Geometry check sheet. Reference: the model listing, model coordinates, mm. Face numbers are marked on the shaded views. A direction names the side the tool comes from. Round coordinates to 2 decimals unless told otherwise and drop trailing zeros. Write each loop counter-clockwise with the first axis right and the second up, starting at its lowest first coordinate (ties: lowest second). Pieces come first, ordered by that corner, then holes. Notation, with made-up numbers: (29.5, -1.5) -> (35.5, -1.5) arc R34 cw to (35.5, 32.5) -> close; hole circle Ø10 at (-38.5, 31). An arc over 180 degrees is marked (long way). One line per question, with ' | ' between items.
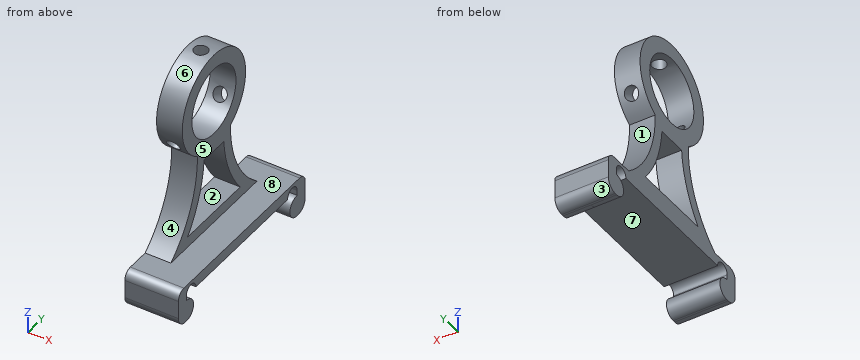
Autodesk Inventor part; units mm, degrees
ref_plane "Work Plane1" through (0, 0, 88) normal (0, 0, 1) x (1, 0, 0)
ref_plane "YZ Plane" through (0, 0, 0) normal (1, 0, 0) x (0, 1, 0)
ref_plane "XZ Plane" through (0, 0, 0) normal (0, 1, 0) x (-1, 0, 0)
sketch "Sketch1" plane through (0, 0, 0) normal (1, 0, 0) x (0, 1, 0)
  line L0 (-46, -7.5) -> (-46, 1)
  line L1 (-42, 5) -> (42, 5)
  line L2 (46, 1) -> (46, -7.5)
  line L3 (-41, -12.5) -> (-39.95, -12.5)
  line L4 (-40.25, -2.509) -> (-40.25, 0)
  line L5 (-40.25, 0) -> (40.25, 0)
  arc A0 (46, 1) -> (42, 5) centre (42, 1) ccw
  arc A1 (-42, 5) -> (-46, 1) centre (-42, 1) ccw
  arc A2 (40.25, 0) -> (33.25, 0) centre (36.75, 0) ccw
  arc A3 (-33.25, 0) -> (-40.25, 0) centre (-36.75, 0) ccw
  line L6 (40.25, 0) -> (40.25, -2.509)
  arc A4 (-39.95, -12.5) -> (-40.25, -2.509) centre (-39.95, -7.5) ccw
  arc A5 (-46, -7.5) -> (-41, -12.5) centre (-41, -7.5) ccw
  circle A6 centre (39.95, -7.5) radius 5
  line L7 (41, -12.5) -> (39.95, -12.5)
  arc A7 (41, -12.5) -> (46, -7.5) centre (41, -7.5) ccw
  circle A8 centre (0, 65) radius 16
  circle A9 centre (0, 65) radius 23
  arc A10 (-31.25, 5) -> (-12, 45.3786) centre (-61.9911, 44.4333) ccw
  arc A11 (12, 45.3786) -> (31.25, 5) centre (61.9911, 44.4333) ccw
  point P0 (0, 0)
  point P1 (-46, -12.5)
  point P2 (-46, 5)
  point P3 (46, 5)
  point P4 (46, -12.5)
  point P5 (0, 0)
  point P6 (-40.25, -1.2545)
  point P7 (40.25, -1.2545)
  point P8 (40.25, -2.509)
  point P9 (0, 5)
  dimension "d71" = 10
  dimension "d2" = 80.5
  dimension "d10" = 92
  dimension "d11" = 5
  dimension "d52" = 4
  dimension "d53" = 7
  dimension "d54" = 7
  dimension "d67" = 10
  dimension "d68" = 7.5
  dimension "d69" = 0.3
  dimension "d70" = 5
  dimension "d72" = 0.3
  dimension "d73" = 5
  dimension "d74" = 32
  dimension "d75" = 7
  dimension "d76" = 65
  dimension "d77" = 2
  dimension "d78" = 2
  dimension "d79" = 12
  dimension "d80" = 50
extrude "Extrusion1" add sketch "Sketch1" along normal mid plane 12 contours L0 A1 L1 A0 L2 A7 L7 A6 L6 A2 L5 A3 L4 A4 L3 A5 | A10 A9 A11 L1 | A9 | A6
sketch "Sketch7" plane through (6, 0, 0) normal (1, 0, 0) x (0, 0, -1)
  arc A0 (-45.3786, 12) -> (-5, 31.25) centre (-44.4333, 61.9911) ccw
  arc A1 (-5, -31.25) -> (-45.3786, -12) centre (-44.4333, -61.9911) ccw
  arc A2 (-45.3786, 12) -> (-45.3786, -12) centre (-65, 0) ccw
  line L0 (-45.3786, 12) -> (-45.3786, -12)
  arc A3 (-45.3786, 12) -> (-5, 31.25) centre (-44.4333, 61.9911) ccw
  line L1 (-5, 31.25) -> (-5, -31.25)
  line L2 (0, -33.25) -> (0, 33.25)
  arc A4 (-45.3786, 12) -> (-5, 31.25) centre (-44.4333, 61.9911) ccw
  arc A5 (-5, -31.25) -> (-45.3786, -12) centre (-44.4333, -61.9911) ccw
  arc A6 (-5, -31.25) -> (-45.3786, -12) centre (-44.4333, -61.9911) ccw
  arc A7 (-10, -19.1035) -> (-40.3786, -7.1407) centre (-44.4333, -61.9911) ccw
  line L3 (-40.3786, -7.1407) -> (-40.3786, 7.1407)
  arc A8 (-40.3786, 7.1407) -> (-10, 19.1035) centre (-44.4333, 61.9911) ccw
  line L4 (-10, 19.1035) -> (-10, -19.1035)
  point P0 (0, 0)
  dimension "d81" = 5
extrude "Extrusion4" cut sketch "Sketch7" against normal through all contours A7 L3 A8 L4
sketch "Sketch8" plane through (6, 0, 0) normal (1, 0, 0) x (0, 0, -1)
  line L0 (-40.3786, -7.1407) -> (-40.3786, 7.1407)
  arc A0 (-40.3786, 7.1407) -> (-10, 19.1035) centre (-44.4333, 61.9911) ccw
  line L1 (-10, 19.1035) -> (-10, -19.1035)
  arc A1 (-10, -19.1035) -> (-40.3786, -7.1407) centre (-44.4333, -61.9911) ccw
  arc A2 (0, -33.25) -> (0, -40.25) centre (0, -36.75) ccw
  line L2 (0, -33.25) -> (0, 33.25)
  arc A3 (0, 40.25) -> (0, 33.25) centre (0, 36.75) ccw
  line L3 (0, 40.25) -> (2.509, 40.25)
  arc A4 (2.509, 40.25) -> (12.5, 39.95) centre (7.5, 39.95) ccw
  line L4 (12.5, 39.95) -> (12.5, 41)
  arc A5 (12.5, 41) -> (7.5, 46) centre (7.5, 41) ccw
  line L5 (7.5, 46) -> (-1, 46)
  arc A6 (-1, 46) -> (-5, 42) centre (-1, 42) ccw
  line L6 (-5, 42) -> (-5, 31.25)
  arc A7 (-45.3786, 12) -> (-5, 31.25) centre (-44.4333, 61.9911) ccw
  arc A8 (-45.3786, 12) -> (-45.3786, -12) centre (-65, 0) ccw
  arc A9 (-5, -31.25) -> (-45.3786, -12) centre (-44.4333, -61.9911) ccw
  line L7 (-5, -31.25) -> (-5, -42)
  arc A10 (-5, -42) -> (-1, -46) centre (-1, -42) ccw
  line L8 (-1, -46) -> (7.5, -46)
  arc A11 (7.5, -46) -> (12.5, -41) centre (7.5, -41) ccw
  line L9 (12.5, -41) -> (12.5, -39.95)
  arc A12 (12.5, -39.95) -> (2.509, -40.25) centre (7.5, -39.95) ccw
  line L10 (2.509, -40.25) -> (0, -40.25)
  circle A13 centre (-65, 0) radius 16
  line L11 (-5, 31.25) -> (-5, -31.25)
  point P0 (0, 0)
extrude "Extrusion5" add sketch "Sketch8" along normal blind 13 contours A2 L10 A12 L9 A11 L8 A10 L7 L11 L6 A6 L5 A5 L4 A4 L3 A3 L2
ref_plane "Work Plane1" through (0, 0, 88) normal (0, 0, 1) x (1, 0, 0)
sketch "Sketch9" plane through (0, 0, 88) normal (0, 0, 1) x (1, 0, 0)
  point P0 (0, 0)
  point P1 (0, 0)
hole "Hole4" at (0, 0, 88) direction (0, 0, -1) diameter 6.4 depth 10
pattern_circular "Circular Pattern1" count 3 over 360 about axis through (0, 0, 65) along (1, 0, 0) of "Hole4"
properties part number "Rail-HeNeHolder" material "ABS Plastic"
(1) Sectioned sample at B-B on y = 36.75. Record the cut outline in (x, z), then the cut area to 3 significant figures.
Resolved:
outline: (-6, -11.34) -> (19, -11.34) -> (19, -3.66) -> (-6, -3.66) -> close; (-6, 3.5) -> (19, 3.5) -> (19, 5) -> (-6, 5) -> close | area: 230 mm2
(2) Material ranges on line 1 (X direction, y = 0, z = 84.75); line 2 (Z direction, x = -2, y = 0); line 3 (Z direction, x = 14.75, y = -12), recorded low to high.
Resolved:
line 1: x = -6 to -3.2, 3.2 to 6 | line 2: z = 0 to 10, 40.38 to 49 | line 3: z = 0 to 5
(3) Go/stop test with flat-tipped pins: pin 1 (10 mm diameter, centred on x = 13.5, z = 68.5, fed in from -Y); pin 2 (8 mm diameter, centred on x = 8.5, z = 31, fed in from +Y); pin 3 (3 mm diameter, centred on x = 1, z = 15.5, fed in from -Y); pin 4 (7.5 mm diameter, centred on x = 0, y = 0, fed in from -Z). Record where each tip stops, or that it passes through.
Resolved:
pin 1: passes through | pin 2: stops at y = 14.81 | pin 3: stops at y = -22.32 | pin 4: stops at z = 0
(4) Sectioned sample at D-D on x = 1.25. Count the separate pieces of the cut face and the enclosed holes in it, then the cut area to 3 significant figures.
Resolved:
separate pieces: 3 | enclosed holes: 1 | area: 2,050 mm2
(5) Draft check along Y on the marked faces 6, 7 and 8. Enter one of: +Y half, -Y half, draft (parallel to the pull), parting line (faces both ways), or undercut.
Resolved:
face 6: parting line | face 7: undercut | face 8: draft
(6) Access from +Z, -Z, +X, -X, +Y, -Y to the whole of each face (thin tool, end or side, straight path). Record for the marked faces 1, 2, 3, 4 and 5.
Resolved:
face 1: +X, -X, +Y | face 2: +X, -X | face 3: -Z, +X, -X, +Y | face 4: +X, -X, -Y | face 5: +Z, +X, +Y, -Y
(7) Sectioned sample at A-A on z = 15. Record the cut outline in (x, y).
Resolved:
outline: (-6, -21.57) -> (6, -21.57) -> (6, -15.53) -> (-6, -15.53) -> close; (-6, 15.53) -> (6, 15.53) -> (6, 21.57) -> (-6, 21.57) -> close
(8) Sectioned sample at C-C on x = 10.75. Record the cut outline in (y, z), then the cut area to 3 significant figures.
Resolved:
outline: (-46, -7.5) arc R5 ccw to (-41, -12.5) -> (-39.95, -12.5) arc R5 ccw (long way) to (-40.25, -2.51) -> (-40.25, 0) arc R3.5 cw to (-33.25, 0) -> (33.25, 0) arc R3.5 cw to (40.25, 0) -> (40.25, -2.51) arc R5 ccw (long way) to (39.95, -12.5) -> (41, -12.5) arc R5 ccw to (46, -7.5) -> (46, 1) arc R4 ccw to (42, 5) -> (-42, 5) arc R4 ccw to (-46, 1) -> close | area: 632 mm2
